```python
from build123d import *

# Parameters (mm, degrees)
SKETCH1_R           = 14.351
BOSS_EXTRUDE1_DEPTH = 29.2608
SKETCH2_R           = 22.6949
BOSS_EXTRUDE2_DEPTH = 42.9006
SKETCH3_R           = 49.2379
BOSS_EXTRUDE3_DEPTH = 679.704
SKETCH4_R           = 49.2379
SKETCH4_R_2         = 41.6179
BOSS_EXTRUDE4_DEPTH = 29.9212
SKETCH5_R           = 4.64185
CUT_EXTRUDE1_DEPTH  = 74.99858
SKETCH6_R           = 50.5079
BOSS_EXTRUDE5_DEPTH = 12.7
SKETCH9_R           = 38.900000051
SKETCH8_R           = 44.621320206
FILLET1_R           = 0.762


with BuildPart() as part:
    # Sketch1 → Boss-Extrude1 (new body)
    with BuildSketch(Plane(origin=(0, 0, 0), x_dir=(1, 0, 0), z_dir=(0, 1, 0))):
        Circle(SKETCH1_R)
    extrude(amount=-BOSS_EXTRUDE1_DEPTH)

    # Sketch2 → Boss-Extrude2 (add)
    with BuildSketch(Plane.XZ.offset(29.2608)):
        Circle(SKETCH2_R)
    extrude(amount=BOSS_EXTRUDE2_DEPTH)

    # Sketch3 → Boss-Extrude3 (add)
    with BuildSketch(Plane.XZ.offset(72.1614)):
        Circle(SKETCH3_R)
    extrude(amount=BOSS_EXTRUDE3_DEPTH)

    # Sketch4 → Boss-Extrude4 (add)
    with BuildSketch(Plane(origin=(0, -72.1614, 0), x_dir=(1, 0, 0), z_dir=(0, 1, 0))):
        Circle(SKETCH4_R)
        Circle(SKETCH4_R_2, mode=Mode.SUBTRACT)
    extrude(amount=BOSS_EXTRUDE4_DEPTH)

    # Sketch5 → Cut-Extrude1 (cut)
    with BuildSketch(Plane(origin=(0, 0, 0), x_dir=(1, 0, 0), z_dir=(0, 1, 0))):
        Circle(SKETCH5_R)
    extrude(amount=-CUT_EXTRUDE1_DEPTH, mode=Mode.SUBTRACT)

    # Sketch6 → Boss-Extrude5 (add)
    with BuildSketch(Plane.XZ.offset(751.8654)):
        Circle(SKETCH6_R)
    extrude(amount=BOSS_EXTRUDE5_DEPTH)

    # Sketch9 → Cut-Loft1 section 0
    with BuildSketch(Plane(origin=(0, -747.837378846, 0), x_dir=(-1, 0, 0), z_dir=(0, -1, 0))):
        Circle(SKETCH9_R)
    # Sketch8 → Cut-Loft1 section 1
    with BuildSketch(Plane.XZ.offset(764.5654)):
        Circle(SKETCH8_R)
    loft(mode=Mode.SUBTRACT)

    # Fillet1
    fillet1_edges = [part.edges().sort_by_distance(p)[0] for p in [
        (-14.351, 0, 0),
        (-14.351, -29.2608, 0),
        (-22.6949, -29.2608, 0),
        (-22.6949, -72.1614, 0),
    ]]
    fillet(fillet1_edges, radius=FILLET1_R)


solid = part.part
```
Here's how the part is built. I have some questions about the finished solid (model axes, mm). A direction names the side the tool comes from. Coordinates: 2 decimals unless noted, no trailing zeros. Order: outer loops, then holes, each group sorted by start corner. A loop starts at its lowest first (then second) coordinate and runs counter-clockwise, first axis right, second up.
1) Will these pins go through, and if not, where does the flat tip stop? pin 1 (12 mm diameter, centred on x = 23.5, y = -622, fed in from -Z); pin 2 (3 mm diameter, centred on x = -25.5, z = 15.5, fed in from -Y); pin 3 (12 mm diameter, centred on y = -315, z = 26, fed in from -X).
2) We'd pull the mould along Z, two halves only. Please class faces 4 (the face through (-37.445, -748.884, -11.792)), 5 (the face through (-11.2, -42.24, -40.3)), 6 (the face through (-10.949, -758.127, -49.307)): +Z half, -Z half, draft (parallel to the pull), parting line (faces both ways), or undercut.
3) Imagine slicing it at A-A on y = -324.5. List the corners of the cut face in (x, z) for me, and give its area (3 significant figures).
4) I need wall thicknesses on line 1 (Z direction, x = 0, y = -61.5); line 2 (Z direction, x = 0, y = -20.5); line 3 (Y direction, x = 9, z = -35). Which ranges of each line are inside material? Lowest first, please.
5) Which directions (+Z, -Z, +X, -X, +Y, -Y) give clear straight access to the entire face, cutting with the end or side of a thin tool? Please do faces 1 (the face through (0, -764.565, -45)), 2 (the face through (-3.11, -14.44, 14.01)), 3 (the face through (1, -747.837, -1)).
Response values:
1. pin 1: stops at z = -46.02
1. pin 2: stops at y = -747.84
1. pin 3: stops at x = -44.99
2. face 4: undercut
2. face 5: draft
2. face 6: parting line
3. outline: circle Ø98.48 at (0, 0)
3. area: 7,620 mm2
4. line 1: z = -49.24 to -41.62, -22.69 to -4.64, 4.64 to 22.69, 41.62 to 49.24
4. line 2: z = -14.35 to -4.64, 4.64 to 14.35
4. line 3: y = -747.84 to -72.16
5. face 1: +Z, -Z, +X, -X, -Y
5. face 2: +Y
5. face 3: -Y
